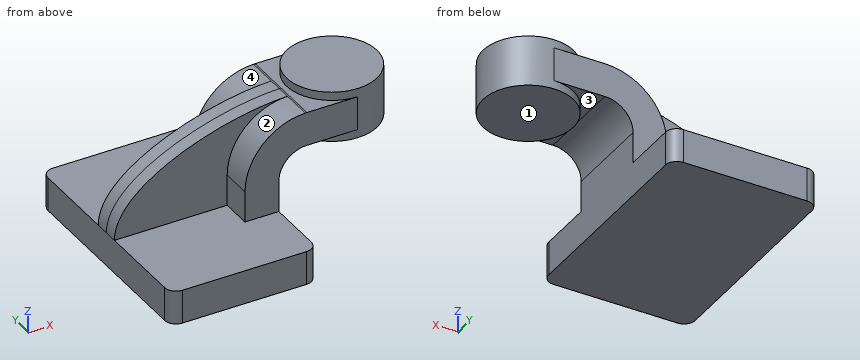
```python
from build123d import *

# Parameters (mm, degrees)
F1_DEPTH  = 63.5
F2_DEPTH  = 25.4
F3_DEPTH  = 7.9375
F2_FACE_W = 50.8
F2_FACE_H = 19.05
F4_DEPTH  = 25.4
F6_R      = 6.35


with BuildPart() as f1:
    # F0 (on Front) → F1 (new body, symmetric)
    with BuildSketch(Plane.XZ):
        Polygon((-41.275, -9.525), (41.275, -9.525), (41.275, 9.525), (22.225, 9.525), (-41.275, 9.525), align=None)
    extrude(amount=F1_DEPTH, both=True)

    # F0 (on Front) → F2 (join, symmetric)
    with BuildSketch(Plane.XZ):
        with BuildLine():
            Line((22.225, 9.525), (41.275, 9.525))
            Line((41.275, 9.525), (41.275, 27.0002))
            ThreePointArc((41.275, 27.0002), (45.92468, 38.22552), (57.15, 42.8752))
            Line((57.15, 42.8752), (60.325, 42.8752))
            Line((60.325, 42.8752), (60.325, 61.9252))
            Line((60.325, 61.9252), (57.15, 61.9252))
            add(Edge.make_bspline(
                [(56.246263, 61.913505), (56.548882, 61.918749), (56.850141, 61.92265), (57.15, 61.9252)],
                knots=[110.625514, 110.625514, 110.625514, 110.625514, 111.504536, 111.504536, 111.504536, 111.504536], degree=3))
            ThreePointArc((56.246263, 61.913505), (32.136817, 51.374291), (22.225, 27.0002))
            Line((22.225, 27.0002), (22.225, 9.525))
        make_face()
    extrude(amount=F2_DEPTH, both=True)

    # F0 (on Front) → F3 (join, symmetric)
    with BuildSketch(Plane.XZ):
        with BuildLine():
            add(Edge.make_bspline(
                [(-41.275, 9.525), (-41.458409, 39.311917), (18.161459, 61.253523), (56.246263, 61.913505)],
                knots=[0, 0, 0, 0, 110.625514, 110.625514, 110.625514, 110.625514], degree=3))
            Line((-41.275, 9.525), (22.225, 9.525))
            Line((22.225, 9.525), (22.225, 27.0002))
            ThreePointArc((22.225, 27.0002), (32.136817, 51.374291), (56.246263, 61.913505))
        make_face()
    extrude(amount=F3_DEPTH, both=True)

    # F2_face (on face) → F4 (join, through all)
    with BuildSketch(Plane(origin=(60.325, 0, 52.4002), x_dir=(0, 1, 0), z_dir=(1, 0, 0))):
        Rectangle(F2_FACE_W, F2_FACE_H)
    extrude(amount=F4_DEPTH)

    # F0 (on Front) → F5 (revolve)
    with BuildSketch(Plane.XZ):
        Polygon((85.725, 61.9252), (85.725, 42.8752), (85.725, 38.1), (111.125, 38.1), (111.125, 66.675), (85.725, 66.675), align=None)
    revolve(axis=Axis((85.725, 0, 52.3875), (0, 0, 1)))

    # F6
    f6_edges = [f1.edges().sort_by_distance(p)[0] for p in [
        (41.275, 63.5, 0),
        (-41.275, 63.5, 0),
        (-41.275, -63.5, 0),
        (41.275, -63.5, 0),
    ]]
    fillet(f6_edges, radius=F6_R)


solid = f1.part
```
CAD build for the part. Positions are in the model's coordinates, mm. Face numbers are marked on the shaded views. A direction names the side the tool comes from. Round coordinates to 2 decimals unless told otherwise and drop trailing zeros. Order: outer loops, then holes, each group sorted by start corner. A loop starts at its lowest first (then second) coordinate and runs counter-clockwise, first axis right, second up.
Q1. Wall check: L1, parallel to Z at x = 9, y = -17.5 (3 decimals); L2, parallel to Y at x = 44, z = 51; L3, parallel to Z at x = 76.5, y = -11.5 (3 decimals). Give the ranges that are in metal, low to high.
Q2. Drop flat-ended pins along their axis: pin 1 (1.5 mm diameter, centred on x = 36.5, y = 18.5, fed in from +Z); pin 2 (5 mm diameter, centred on y = 15, z = 17.5, fed in from -X) (3 decimals); pin 3 (10 mm diameter, centred on x = 56, y = -13.5, fed in from -Z); pin 4 (15.5 mm diameter, centred on x = 60.5, z = 25.5, fed in from +Y). Give the stop position or say it passes through.
Q3. Slice it at D-D (x = 97). Write the cut outline in (y, z) (3 decimals), and give its area (3 significant figures).
Q4. Slice it at B-B (z = 7). Write the cut outline in (x, y) (3 decimals).
Q5. Slice it at C-C (y = 53.5). Write the cut outline in (x, z) (3 decimals), and give its area (3 significant figures).
Q6. Which spindle directions (+Z, -Z, +X, -X, +Y, -Y) get a long thin tool onto all of the face, cutting with end or side? Do the marked faces 1, 2, 3 and 4. Say none if no direction does.
Q7. Slice it at A-A (x = 69.5). Write the cut outline in (y, z) (1 decimal).
Results below:
1. L1: z = -9.525 to 9.525
1. L2: y = -25.4 to 25.4
1. L3: z = 38.1 to 66.675
2. pin 1: stops at z = 55.7
2. pin 2: stops at x = 22.225
2. pin 3: stops at z = 41.64
2. pin 4: passes through
3. outline: (-22.76, 38.1) - (22.76, 38.1) - (22.76, 66.675) - (-22.76, 66.675) - close
3. area: 1,300 mm2
4. outline: (-41.275, -57.15) arc R6.35 ccw to (-34.925, -63.5) - (34.925, -63.5) arc R6.35 ccw to (41.275, -57.15) - (41.275, 57.15) arc R6.35 ccw to (34.925, 63.5) - (-34.925, 63.5) arc R6.35 ccw to (-41.275, 57.15) - close
5. outline: (-41.275, -9.525) - (41.275, -9.525) - (41.275, 9.525) - (-41.275, 9.525) - close
5. area: 1,570 mm2
6. face 1: -Z, +X, +Y, -Y
6. face 2: +Z, -X, -Y
6. face 3: -Z
6. face 4: +Z, -X, +Y
7. outline: (-25.4, 42.9) - (-19.5, 42.9) - (-19.5, 38.1) - (19.5, 38.1) - (19.5, 42.9) - (25.4, 42.9) - (25.4, 61.9) - (19.5, 61.9) - (19.5, 66.7) - (-19.5, 66.7) - (-19.5, 61.9) - (-25.4, 61.9) - close
